```python
from build123d import *

# Parameters (mm, degrees)
SKETCH1_W           = 15.24
SKETCH1_H           = 25.4
BOSS_EXTRUDE1_DEPTH = 5.08
FILLET1_R           = 2.54
SKETCH2_R           = 3.175
BOSS_EXTRUDE2_DEPTH = 6.35
SKETCH3_W           = 5.08
SKETCH3_H           = 10.16
BOSS_EXTRUDE3_DEPTH = 5.08
SKETCH4_W           = 7.62
SKETCH4_H           = 12.7
BOSS_EXTRUDE4_DEPTH = 25.4
FILLET2_R           = 2.54
FILLET3_R           = 3.81
SKETCH5_R           = 1.905
BOSS_EXTRUDE5_DEPTH = 1.27
BOSS_EXTRUDE6_DEPTH = 25.4
FILLET4_R           = 1.27
SKETCH7_W           = 5.588
SKETCH7_H           = 21.59
CUT_EXTRUDE1_DEPTH  = 1.016
FILLET5_R           = 0.254
CUT_EXTRUDE2_REACH  = 52.512
SKETCH8_R           = 4.445
FILLET6_R           = 0.635
SKETCH9_W           = 25.4
SKETCH9_H           = 50.8
CUT_EXTRUDE3_DEPTH  = 22.86
SKETCH10_R          = 3.175
CUT_EXTRUDE4_DEPTH  = 12.7


# Some blends are built 0.0001 mm under size
with BuildPart() as part:
    # Sketch1 → Boss-Extrude1 (new, symmetric)
    with BuildSketch(Plane(origin=(0, 0, 0), x_dir=(0, 0, -1), z_dir=(1, 0, 0))):
        Rectangle(SKETCH1_W, SKETCH1_H)
    extrude(amount=BOSS_EXTRUDE1_DEPTH, both=True)

    # Fillet1
    fillet1_edges = [part.edges().sort_by_distance(p)[0] for p in [
        (5.08, 0, 7.62),
        (5.08, -12.7, 0),
        (5.08, 0, -7.62),
        (-5.08, -12.7, 0),
        (-5.08, 0, 7.62),
        (-5.08, 12.7, 0),
        (-5.08, 0, -7.62),
        (5.08, 12.7, 0),
        (0, -12.7, -7.62),
        (0, -12.7, 7.62),
        (0, 12.7, 7.62),
        (0, 12.7, -7.62),
    ]]
    fillet(fillet1_edges, radius=FILLET1_R)

    # Sketch2 → Boss-Extrude2 (add)
    with BuildSketch(Plane(origin=(5.08, 0, 0), x_dir=(0, 0, -1), z_dir=(1, 0, 0))):
        with Locations(Location((0, 6.985, 0), (0, 0, 90))):
            Circle(SKETCH2_R)
        with Locations(Location((0, -6.985, 0), (0, 0, 270))):
            Circle(SKETCH2_R)
    boss_extrude2 = extrude(amount=BOSS_EXTRUDE2_DEPTH)

    # Mirror1: Boss-Extrude2 across plane
    add(boss_extrude2.mirror(Plane(origin=(0, 0, 0), x_dir=(0, 0, 1), z_dir=(1, 0, 0))))

    # Sketch3 → Boss-Extrude3 (add)
    with BuildSketch(Plane(origin=(0, 12.7, 0), x_dir=(1, 0, 0), z_dir=(0, 1, 0))):
        Rectangle(SKETCH3_W, SKETCH3_H)
    extrude(amount=BOSS_EXTRUDE3_DEPTH)

    # Sketch4 → Boss-Extrude4 (add)
    with BuildSketch(Plane(origin=(0, 17.78, 0), x_dir=(1, 0, 0), z_dir=(0, 1, 0))):
        Rectangle(SKETCH4_W, SKETCH4_H)
    extrude(amount=BOSS_EXTRUDE4_DEPTH)

    # Fillet2
    # the kernel refuses this fillet: 2.54 mm, written as the material it takes off along each edge
    with BuildSketch(Plane(origin=(10.16, 17.78, -6.35), x_dir=(0, 0, 1), z_dir=(-1, 0, 0))) as fillet2_piece_1_section:
        with BuildLine():
            CenterArc((FILLET2_R, FILLET2_R), FILLET2_R, 180, 90)
            Line((0, FILLET2_R), (0, 0))
            Line((0, 0), (FILLET2_R, 0))
        make_face()
    fillet2_piece_1 = extrude(amount=20.32, mode=Mode.PRIVATE)
    fillet2_piece_1 = split(fillet2_piece_1, bisect_by=Plane(origin=(6.35, 17.840981289, -5.08), z_dir=(0, 0, 1)), keep=Keep.TOP, mode=Mode.PRIVATE)
    fillet2_piece_1 = split(fillet2_piece_1, bisect_by=Plane(origin=(2.54, 17.840981289, -4.665343007), z_dir=(1, 0, 0)), keep=Keep.TOP, mode=Mode.PRIVATE)
    add(fillet2_piece_1, mode=Mode.SUBTRACT)
    with BuildSketch(Plane(origin=(10.16, 17.78, -6.35), x_dir=(0, 0, 1), z_dir=(-1, 0, 0))) as fillet2_piece_2_section:
        with BuildLine():
            CenterArc((FILLET2_R, FILLET2_R), FILLET2_R, 180, 90)
            Line((0, FILLET2_R), (0, 0))
            Line((0, 0), (FILLET2_R, 0))
        make_face()
    fillet2_piece_2 = extrude(amount=20.32, mode=Mode.PRIVATE)
    fillet2_piece_2 = split(fillet2_piece_2, bisect_by=Plane(origin=(6.35, 18.428004952, -5.08), z_dir=(0, 0, -1)), keep=Keep.TOP, mode=Mode.PRIVATE)
    fillet2_piece_2 = split(fillet2_piece_2, bisect_by=Plane(origin=(2.54, 18.428004952, -5.932444919), z_dir=(1, 0, 0)), keep=Keep.TOP, mode=Mode.PRIVATE)
    add(fillet2_piece_2, mode=Mode.SUBTRACT)
    with BuildSketch(Plane(origin=(10.16, 17.78, -6.35), x_dir=(0, 0, 1), z_dir=(-1, 0, 0))) as fillet2_piece_3_section:
        with BuildLine():
            CenterArc((FILLET2_R, FILLET2_R), FILLET2_R, 180, 90)
            Line((0, FILLET2_R), (0, 0))
            Line((0, 0), (FILLET2_R, 0))
        make_face()
    fillet2_piece_3 = extrude(amount=20.32, mode=Mode.PRIVATE)
    fillet2_piece_3 = split(fillet2_piece_3, bisect_by=Plane(origin=(0, 18.428004952, -5.08), z_dir=(0, 0, -1)), keep=Keep.TOP, mode=Mode.PRIVATE)
    fillet2_piece_3 = split(fillet2_piece_3, bisect_by=Plane(origin=(-2.54, 18.428004952, -5.932444919), z_dir=(1, 0, 0)), keep=Keep.TOP, mode=Mode.PRIVATE)
    fillet2_piece_3 = split(fillet2_piece_3, bisect_by=Plane(origin=(2.54, 18.428004952, -5.932444919), z_dir=(-1, 0, 0)), keep=Keep.TOP, mode=Mode.PRIVATE)
    add(fillet2_piece_3, mode=Mode.SUBTRACT)
    with BuildSketch(Plane(origin=(10.16, 17.78, -6.35), x_dir=(0, 0, 1), z_dir=(-1, 0, 0))) as fillet2_piece_4_section:
        with BuildLine():
            CenterArc((FILLET2_R, FILLET2_R), FILLET2_R, 180, 90)
            Line((0, FILLET2_R), (0, 0))
            Line((0, 0), (FILLET2_R, 0))
        make_face()
    fillet2_piece_4 = extrude(amount=20.32, mode=Mode.PRIVATE)
    fillet2_piece_4 = split(fillet2_piece_4, bisect_by=Plane(origin=(-6.35, 17.840981289, -5.08), z_dir=(0, 0, 1)), keep=Keep.TOP, mode=Mode.PRIVATE)
    fillet2_piece_4 = split(fillet2_piece_4, bisect_by=Plane(origin=(-2.54, 17.840981289, -4.665343007), z_dir=(-1, 0, 0)), keep=Keep.TOP, mode=Mode.PRIVATE)
    add(fillet2_piece_4, mode=Mode.SUBTRACT)
    with BuildSketch(Plane(origin=(10.16, 17.78, -6.35), x_dir=(0, 0, 1), z_dir=(-1, 0, 0))) as fillet2_piece_5_section:
        with BuildLine():
            CenterArc((FILLET2_R, FILLET2_R), FILLET2_R, 180, 90)
            Line((0, FILLET2_R), (0, 0))
            Line((0, 0), (FILLET2_R, 0))
        make_face()
    fillet2_piece_5 = extrude(amount=20.32, mode=Mode.PRIVATE)
    fillet2_piece_5 = split(fillet2_piece_5, bisect_by=Plane(origin=(-6.35, 18.428004952, -5.08), z_dir=(0, 0, -1)), keep=Keep.TOP, mode=Mode.PRIVATE)
    fillet2_piece_5 = split(fillet2_piece_5, bisect_by=Plane(origin=(-2.54, 18.428004952, -5.932444919), z_dir=(-1, 0, 0)), keep=Keep.TOP, mode=Mode.PRIVATE)
    add(fillet2_piece_5, mode=Mode.SUBTRACT)
    with BuildSketch(Plane(origin=(-10.16, 17.78, 6.35), x_dir=(0, 1, 0), z_dir=(1, 0, 0))) as fillet2_piece_6_section:
        with BuildLine():
            CenterArc((FILLET2_R, -FILLET2_R), FILLET2_R, 90, 90)
            Line((0, -FILLET2_R), (0, 0))
            Line((0, 0), (FILLET2_R, 0))
        make_face()
    fillet2_piece_6 = extrude(amount=20.32, mode=Mode.PRIVATE)
    fillet2_piece_6 = split(fillet2_piece_6, bisect_by=Plane(origin=(-2.54, 18.428004952, 5.932444919), z_dir=(-1, 0, 0)), keep=Keep.TOP, mode=Mode.PRIVATE)
    fillet2_piece_6 = split(fillet2_piece_6, bisect_by=Plane(origin=(-6.35, 18.428004952, 5.08), z_dir=(0, 0, 1)), keep=Keep.TOP, mode=Mode.PRIVATE)
    add(fillet2_piece_6, mode=Mode.SUBTRACT)
    with BuildSketch(Plane(origin=(-10.16, 17.78, 6.35), x_dir=(0, 1, 0), z_dir=(1, 0, 0))) as fillet2_piece_7_section:
        with BuildLine():
            CenterArc((FILLET2_R, -FILLET2_R), FILLET2_R, 90, 90)
            Line((0, -FILLET2_R), (0, 0))
            Line((0, 0), (FILLET2_R, 0))
        make_face()
    fillet2_piece_7 = extrude(amount=20.32, mode=Mode.PRIVATE)
    fillet2_piece_7 = split(fillet2_piece_7, bisect_by=Plane(origin=(-2.54, 17.840981289, 4.665343007), z_dir=(-1, 0, 0)), keep=Keep.TOP, mode=Mode.PRIVATE)
    fillet2_piece_7 = split(fillet2_piece_7, bisect_by=Plane(origin=(-6.35, 17.840981289, 5.08), z_dir=(0, 0, -1)), keep=Keep.TOP, mode=Mode.PRIVATE)
    add(fillet2_piece_7, mode=Mode.SUBTRACT)
    with BuildSketch(Plane(origin=(-10.16, 17.78, 6.35), x_dir=(0, 1, 0), z_dir=(1, 0, 0))) as fillet2_piece_8_section:
        with BuildLine():
            CenterArc((FILLET2_R, -FILLET2_R), FILLET2_R, 90, 90)
            Line((0, -FILLET2_R), (0, 0))
            Line((0, 0), (FILLET2_R, 0))
        make_face()
    fillet2_piece_8 = extrude(amount=20.32, mode=Mode.PRIVATE)
    fillet2_piece_8 = split(fillet2_piece_8, bisect_by=Plane(origin=(-2.54, 18.428004952, 5.932444919), z_dir=(1, 0, 0)), keep=Keep.TOP, mode=Mode.PRIVATE)
    fillet2_piece_8 = split(fillet2_piece_8, bisect_by=Plane(origin=(0, 18.428004952, 5.08), z_dir=(0, 0, 1)), keep=Keep.TOP, mode=Mode.PRIVATE)
    fillet2_piece_8 = split(fillet2_piece_8, bisect_by=Plane(origin=(2.54, 18.428004952, 5.932444919), z_dir=(-1, 0, 0)), keep=Keep.TOP, mode=Mode.PRIVATE)
    add(fillet2_piece_8, mode=Mode.SUBTRACT)
    with BuildSketch(Plane(origin=(-10.16, 17.78, 6.35), x_dir=(0, 1, 0), z_dir=(1, 0, 0))) as fillet2_piece_9_section:
        with BuildLine():
            CenterArc((FILLET2_R, -FILLET2_R), FILLET2_R, 90, 90)
            Line((0, -FILLET2_R), (0, 0))
            Line((0, 0), (FILLET2_R, 0))
        make_face()
    fillet2_piece_9 = extrude(amount=20.32, mode=Mode.PRIVATE)
    fillet2_piece_9 = split(fillet2_piece_9, bisect_by=Plane(origin=(6.35, 18.428004952, 5.08), z_dir=(0, 0, 1)), keep=Keep.TOP, mode=Mode.PRIVATE)
    fillet2_piece_9 = split(fillet2_piece_9, bisect_by=Plane(origin=(2.54, 18.428004952, 5.932444919), z_dir=(1, 0, 0)), keep=Keep.TOP, mode=Mode.PRIVATE)
    add(fillet2_piece_9, mode=Mode.SUBTRACT)
    with BuildSketch(Plane(origin=(-10.16, 17.78, 6.35), x_dir=(0, 1, 0), z_dir=(1, 0, 0))) as fillet2_piece_10_section:
        with BuildLine():
            CenterArc((FILLET2_R, -FILLET2_R), FILLET2_R, 90, 90)
            Line((0, -FILLET2_R), (0, 0))
            Line((0, 0), (FILLET2_R, 0))
        make_face()
    fillet2_piece_10 = extrude(amount=20.32, mode=Mode.PRIVATE)
    fillet2_piece_10 = split(fillet2_piece_10, bisect_by=Plane(origin=(6.35, 17.840981289, 5.08), z_dir=(0, 0, -1)), keep=Keep.TOP, mode=Mode.PRIVATE)
    fillet2_piece_10 = split(fillet2_piece_10, bisect_by=Plane(origin=(2.54, 17.840981289, 4.665343007), z_dir=(1, 0, 0)), keep=Keep.TOP, mode=Mode.PRIVATE)
    add(fillet2_piece_10, mode=Mode.SUBTRACT)

    # Fillet3
    fillet3_edges = [part.edges().sort_by_distance(p)[0] for p in [
        (3.81, 43.18, 0),
        (0, 43.18, -6.35),
        (-3.81, 43.18, 0),
        (0, 43.18, 6.35),
    ]]
    fillet(fillet3_edges, radius=FILLET3_R - 0.0001)  # a hair under: the kernel refuses the full size

    # Sketch5 → Boss-Extrude5 (add)
    with BuildSketch(Plane(origin=(0, 0, -6.35), x_dir=(-1, 0, 0), z_dir=(0, 0, -1))):
        with Locations(Location((0, 32.385, 0), (0, 0, 180))):
            Circle(SKETCH5_R)
        with Locations(Location((0, 25.4, 0), (0, 0, 180))):
            Circle(SKETCH5_R)
    extrude(amount=BOSS_EXTRUDE5_DEPTH)

    # Sketch6 → Boss-Extrude6 (add)
    with BuildSketch(Plane(origin=(0, 21.59, 0), x_dir=(1, 0, 0), z_dir=(0, 1, 0))):
        with BuildLine():
            Line((-3.81, 10.541), (3.81, 10.541))
            ThreePointArc((3.81, 10.541), (5.588, 8.763), (3.81, 6.985))
            Line((3.81, 6.985), (-3.81, 6.985))
            ThreePointArc((-3.81, 6.985), (-5.588, 8.763), (-3.81, 10.541))
        make_face()
    extrude(amount=BOSS_EXTRUDE6_DEPTH)

    # Fillet4
    fillet4_edges = [part.edges().sort_by_distance(p)[0] for p in [
        (0, 21.59, -6.985),
        (-5.588, 21.59, -8.763),
        (5.588, 21.59, -8.763),
        (0, 21.59, -10.541),
        (-5.588, 46.99, -8.763),
        (0, 46.99, -6.985),
        (5.588, 46.99, -8.763),
        (0, 46.99, -10.541),
    ]]
    fillet(fillet4_edges, radius=FILLET4_R)

    # Sketch7 → Cut-Extrude1 (cut)
    with BuildSketch(Plane(origin=(0, 0, -10.541), x_dir=(-1, 0, 0), z_dir=(0, 0, -1))):
        with Locations((0, 34.29)):
            Rectangle(SKETCH7_W, SKETCH7_H)
    extrude(amount=-CUT_EXTRUDE1_DEPTH, mode=Mode.SUBTRACT)

    # Fillet5
    fillet5_edges = [part.edges().sort_by_distance(p)[0] for p in [
        (-2.794, 34.29, -10.541),
        (0, 45.085, -10.541),
        (2.794, 34.29, -10.541),
        (0, 23.495, -10.541),
    ]]
    fillet(fillet5_edges, radius=FILLET5_R)

    # Sketch8 → Cut-Extrude2 (cut, up to next)
    with BuildSketch(Plane(origin=(3.81, 0, 0), x_dir=(0, 0, -1), z_dir=(1, 0, 0)), mode=Mode.PRIVATE) as cut_extrude2_sk1:
        with Locations((0, 33.02)):
            Circle(SKETCH8_R)
    cut_extrude2_tool1 = extrude(cut_extrude2_sk1.sketch, amount=-CUT_EXTRUDE2_REACH, mode=Mode.PRIVATE) & part.part
    add(cut_extrude2_tool1.solids().sort_by_distance((3.81, 33.02, 0))[0], mode=Mode.SUBTRACT)

    # Fillet6
    fillet6_edges = [part.edges().sort_by_distance(p)[0] for p in [
        (11.43, 3.81, 0),
        (11.43, -3.81, 0),
        (-11.43, 3.81, 0),
        (-11.43, -3.81, 0),
    ]]
    fillet(fillet6_edges, radius=FILLET6_R)

    # Sketch9 → Cut-Extrude3 (cut)
    with BuildSketch(Plane(origin=(11.43, 0, 0), x_dir=(0, 0, -1), z_dir=(1, 0, 0))):
        with Locations((0, 38.1)):
            Rectangle(SKETCH9_W, SKETCH9_H)
    extrude(amount=-CUT_EXTRUDE3_DEPTH, mode=Mode.SUBTRACT)

    # Sketch10 → Cut-Extrude4 (cut)
    with BuildSketch(Plane(origin=(0, 12.7, 0), x_dir=(1, 0, 0), z_dir=(0, 1, 0))):
        with Locations(Location((0, 0, 0), (0, 0, 270))):
            Circle(SKETCH10_R)
    extrude(amount=-CUT_EXTRUDE4_DEPTH, mode=Mode.SUBTRACT)


solid = part.part
```
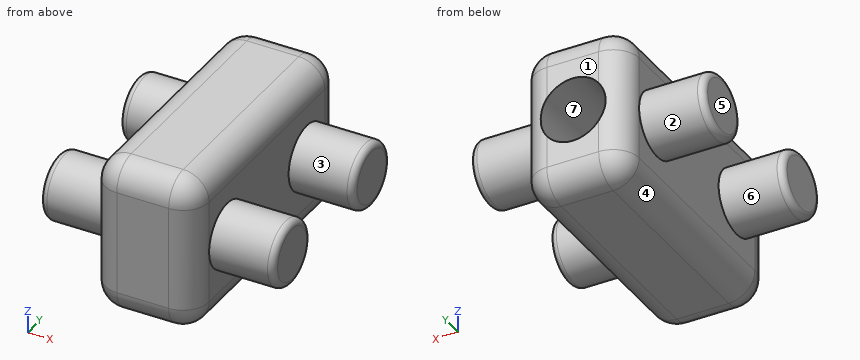
The listing builds one solid part. Answer for the finished solid, in the listing's coordinates (mm). Face numbers are marked on the shaded views. A direction names the side the tool comes from. Round coordinates to 2 decimals unless told otherwise and drop trailing zeros. Write each loop counter-clockwise with the first axis right and the second up, starting at its lowest first coordinate (ties: lowest second). Pieces come first, ordered by that corner, then holes. Notation, with made-up numbers: (-6, 38.5) -> (16, 38.5) arc R18 ccw to (16, 56.5) -> close; hole circle Ø5 at (33, 30.25). An arc over 180 degrees is marked (long way). Answer as a JSON object with one key per item and string values. Group by question number.
Q1. Each of these flat-tipped pins is pushed along its axis until it touches: pin 1 Ø2 at (y, z) = (3.5, 1) entering from -X; pin 2 Ø3 at (x, y) = (-5, -7) entering from +Z; pin 3 Ø1 at (x, y) = (-8, 4.5) entering from -Z. Where does it stop, or does it pass through?
Q2. Section D-D (z = -4.75) is taken. Write down the section's boundary in (x, y).
Q3. Section B-B (x = 0) is taken. Write down the section's boundary in (y, z) (3 decimals), plus the area to 3 significant figures.
Q4. Section A-A (y = 1) is taken. Write down the section's boundary in (x, z) (3 decimals), plus the area to 3 significant figures.
Q5. Determine the mould class of the marked faces 4, 5, 6 and 7 for opening direction Z: pulls with the +Z half, pulls with the -Z half, needs draft (parallel to the pull), parting line crosses it, or undercut.
Q6. Which of the six approach directions +Z, -Z, +X, -X, +Y, -Y give full straight-line access (tool end or side, diameter ignored) to the marked faces 1, 2 and 3?
Q7. Section C-C (x = -6) is taken. Write down the section's boundary in (y, z) (3 decimals), plus the area to 3 significant figures.
Q8. Straight lines are drawn through the part: line 1 along X through (y, z) = (9.25, 0) (3 decimals); line 2 along Y through (x, z) = (1.5, 2.5); line 3 along X through (y, z) = (6.25, -2.5). For each, find the intervals that lie inside material, in ascending order.
Check values:
{
 "1": {"pin 1": "x = -11.42", "pin 2": "z = 7.43", "pin 3": "z = -2.48"},
 "2": {"outline": "(-5.08, -10.16) arc R2.54 ccw to (-2.54, -12.7) -> (2.54, -12.7) arc R2.54 ccw to (5.08, -10.16) -> (5.08, 10.16) arc R2.54 ccw to (2.54, 12.7) -> (-2.54, 12.7) arc R2.54 ccw to (-5.08, 10.16) -> close"},
 "3": {"outline": "(-12.7, -5.08) arc R2.54 ccw to (-10.16, -7.62) -> (10.16, -7.62) arc R2.54 ccw to (12.7, -5.08) -> (12.7, -3.175) -> (0, -3.175) -> (0, 3.175) -> (12.7, 3.175) -> (12.7, 5.08) arc R2.54 ccw to (10.16, 7.62) -> (-10.16, 7.62) arc R2.54 ccw to (-12.7, 5.08) -> close", "area": "301 mm^2"},
 "4": {"outline": "(-5.08, -5.08) arc R2.54 ccw to (-2.54, -7.62) -> (2.54, -7.62) arc R2.54 ccw to (5.08, -5.08) -> (5.08, 5.08) arc R2.54 ccw to (2.54, 7.62) -> (-2.54, 7.62) arc R2.54 ccw to (-5.08, 5.08) -> close; hole circle Ø6.35 at (0, 0)", "area": "118 mm^2"},
 "5": {"face 4": "pulls with the -Z half", "face 5": "needs draft", "face 6": "parting line crosses it", "face 7": "undercut"},
 "6": {"face 1": "+Z, -Z, +X, -X, +Y", "face 2": "-X", "face 3": "+X"},
 "7": {"outline": "circle Ø6.35 at (-6.985, 0); circle Ø6.35 at (6.985, 0)", "area": "63.3 mm^2"},
 "8": {"line 1": "-11.43 to -3.175, 3.175 to 11.43", "line 2": "-12.7 to 0", "line 3": "-11.43 to -1.96, 1.96 to 11.43"}
}
